Here's how the part is built. I have some questions about the finished solid (model axes, mm). A direction names the side the tool comes from. Give positions to 0.01 mm unless a question says otherwise; leave off trailing zeros. Write each loop counter-clockwise with the first axis right and the second up, starting at its lowest first coordinate (ties: lowest second). Pieces come first, ordered by that corner, then holes. Notation, with made-up numbers: (14.25, 9) - (49.25, 9) arc R6 ccw to (49.25, 16) - close; hole circle Ø10 at (62, -36). An arc over 180 degrees is marked (long way). Use a Markdown table: item, result.
Autodesk Inventor part; units mm, degrees
ref_plane "Work Plane1" through (-15.5277, -15.5154, -5.9) normal (0, 0, 1) x (1, 0, 0)
ref_plane "YZ Plane" through (0, 0, 0) normal (1, 0, 0) x (0, 1, 0)
ref_plane "XZ Plane" through (0, 0, 0) normal (0, 1, 0) x (-1, 0, 0)
sketch "Sketch1" plane through (0, 0, 0) normal (0, 0, 1) x (1, 0, 0)
  circle A0 centre (-3.25, -2.15) radius 1
  circle A1 centre (3.25, -2.15) radius 1
  circle A2 centre (-3.25, -2.15) radius 1.1
  circle A3 centre (3.25, -2.15) radius 1.1
  line L0 (-6.45, -0.55) -> (-6.45, -2.95)
  line L1 (6.45, -2.95) -> (6.45, -0.55)
  line L2 (-7.5, 2.95) -> (-10.5, 2.95)
  line L3 (10.5, 2.95) -> (7.5, 2.95)
  line L4 (-7.5, 2.95) -> (7.5, 2.95)
  line L5 (-6.45, 2.95) -> (-6.45, -0.55)
  line L6 (6.45, -0.55) -> (6.45, 2.95)
  line L7 (7.5, 2.95) -> (7.5, -8.05)
  line L8 (-7.5, 2.95) -> (-7.5, -6.5437)
  line L9 (-7.5, 2.95) -> (7.5, 2.95)
  line L10 (7.5, 2.95) -> (7.5, -4.65)
  line L11 (7.5, -4.65) -> (-7.5, -4.65)
  line L12 (-7.5, -4.65) -> (-7.5, 2.95)
  line L13 (-7.4, -4.65) -> (-7.4, 2.95)
  line L14 (7.4, -4.65) -> (7.4, 2.95)
  point P0 (0, 0)
  point P1 (-7.4, 2.95)
  point P2 (7.4, 2.95)
  dimension "d0" = 0.1
  dimension "d1" = 0.1
  dimension "d2" = 7.6
  dimension "d3" = 0.1
  dimension "d4" = 0.1
extrude "Extrusion1" add sketch "Sketch1" along normal blind 3 contours L4 L14 L11 L13
sketch "Sketch2" plane through (0, 0, 0) normal (0, 0, -1) x (-1, 0, 0)
  line L0 (-6.45, -0.55) -> (-6.45, 2.95)
  line L1 (-7.4, -4.65) -> (-7.4, 2.95)
  line L2 (6.45, 2.95) -> (6.45, -0.55)
  line L3 (7.4, 2.95) -> (7.4, -4.65)
  line L4 (-6.55, -0.55) -> (-6.55, 2.95)
  line L5 (6.55, 2.95) -> (6.55, -0.55)
  line L6 (-7.4, 2.95) -> (7.4, 2.95)
  line L7 (7.4, -4.65) -> (-7.4, -4.65)
  line L8 (-7.4, 2.95) -> (-6.55, 2.95)
  line L9 (-6.55, 2.95) -> (-6.55, -4.65)
  line L10 (-6.55, -4.65) -> (-7.4, -4.65)
  line L11 (-7.4, -4.65) -> (-7.4, 2.95)
  line L12 (6.55, 2.95) -> (7.4, 2.95)
  line L13 (7.4, 2.95) -> (7.4, -4.65)
  line L14 (7.4, -4.65) -> (6.55, -4.65)
  line L15 (6.55, -4.65) -> (6.55, 2.95)
  point P0 (0, 0)
  point P1 (6.55, -0.55)
  dimension "d7" = 0.1
  dimension "d8" = 0.1
ref_plane "Work Plane1" through (-15.5277, -15.5154, -5.9) normal (0, 0, 1) x (1, 0, 0)
extrude "Extrusion2" add sketch "Sketch2" along normal up to surface (5.9 mm away) contours L1 L6 L4 L9 L7 | L15 L5 L6 L3 L7
fillet "Fillet1" radius 1.5 2 edges at (7.4, -0.85, 3) (-7.4, -0.85, 3)
properties part number "podkladka_switch"
Item 1: I need wall thicknesses on line 1 along X through (y, z) = (1, -4); line 2 along Z through (x, y) = (-6, 2); line 3 along Y through (x, z) = (-3.25, 0.9). Which ranges of each line are inside material? Lowest first, please. Write a range as [from, to].
Values:
| item | result |
|---|---|
| line 1 | x = [-7.4, -6.55], [6.55, 7.4] |
| line 2 | z = [0, 3] |
| line 3 | y = [-4.65, -3.25], [-1.05, 2.95] |
Item 2: Thinking about a two-plate mould opening in X: for faces 3 (the cylindrical face through (3.84, -3.08, 1.48)), 4 (the flat face through (7.4, -1, -2)), 5 (the flat face through (1.7, -4.65, 0.5)), which applies, +X half, -X half, draft (parallel to the pull), parting line (faces both ways), or undercut?
Values:
| item | result |
|---|---|
| face 3 | undercut |
| face 4 | +X half |
| face 5 | draft |
Item 3: If we section it at D-D, the plane z = 0.25: Write out the boundary of the cut face in (x, y).
Values:
| item | result |
|---|---|
| outline | (-7.4, -4.65) - (7.4, -4.65) - (7.4, 2.95) - (-7.4, 2.95) - close; hole circle Ø2.2 at (-3.25, -2.15); hole circle Ø2.2 at (3.25, -2.15) |
Item 4: If we section it at A-A, the plane z = -3.5: Write out the boundary of the cut face in (x, y).
Values:
| item | result |
|---|---|
| outline | (-7.4, -4.65) - (-6.55, -4.65) - (-6.55, 2.95) - (-7.4, 2.95) - close; (6.55, -4.65) - (7.4, -4.65) - (7.4, 2.95) - (6.55, 2.95) - close |
Item 5: If we section it at C-C, the plane x = 3.25: Write out the boundary of the cut face in (y, z).
Values:
| item | result |
|---|---|
| outline | (-4.65, 0) - (-3.25, 0) - (-3.25, 3) - (-4.65, 3) - close; (-1.05, 0) - (2.95, 0) - (2.95, 3) - (-1.05, 3) - close |
Item 6: For faces 1 (the flat face through (0, -1, 3)), 2 (the flat face through (0, -1, 0)), which set-ups out of +Z, -Z, +X, -X, +Y, -Y let a thin tool reach every point of the face, with its end or its side?
Values:
| item | result |
|---|---|
| face 1 | +Z, +X, -X, +Y, -Y |
| face 2 | -Z, +Y, -Y |
Item 7: If we section it at B-B, the plane y = -2.15: Write out the boundary of the cut face in (x, z).
Values:
| item | result |
|---|---|
| outline | (-7.4, -5.9) - (-6.55, -5.9) - (-6.55, 0) - (-4.35, 0) - (-4.35, 3) - (-5.9, 3) arc R1.5 ccw to (-7.4, 1.5) - close; (-2.15, 0) - (2.15, 0) - (2.15, 3) - (-2.15, 3) - close; (4.35, 0) - (6.55, 0) - (6.55, -5.9) - (7.4, -5.9) - (7.4, 1.5) arc R1.5 ccw to (5.9, 3) - (4.35, 3) - close |
